Can you work these out from the model? Positions are in its coordinate system, mm. Face numbers are marked on the shaded views. Round coordinates to 2 decimals unless told otherwise and drop trailing zeros. Loops run counter-clockwise (first coordinate to the right, second up) from the corner with the lowest first, then second, coordinate; pieces in that order, holes last. Notation, with made-up numbers: (44, 22) -> (59, 22) arc R15 ccw to (59, 40) -> close; hole circle Ø9 at (-31, 39.5). An arc over 180 degrees is marked (long way). Write item = value, one per line.
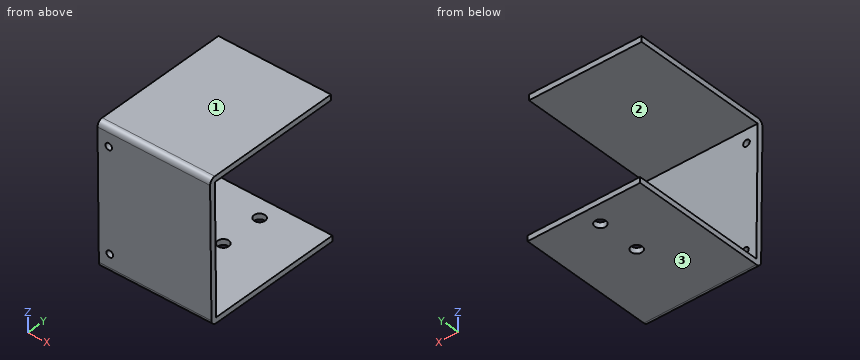
from build123d import *

# Parameters (mm, degrees)
F1_DEPTH = 50.8
F2_R     = 5
F3_DEPTH = 4.9999996097
F4_R     = 3
F5_DEPTH = 128.5401096596


with BuildPart() as f1:
    # F0 (on Right) → F1 (new body, symmetric)
    with BuildSketch(Plane.YZ):
        with BuildLine():
            Line((69.9766400008, 50.951808691), (69.9766400008, 55.9518083008))
            Line((69.9766400008, 55.9518083008), (-51.9620125118, 55.9518083008))
            ThreePointArc((-51.9620125118, 55.9518083008), (-55.5190376607, 54.4657195247), (-56.9616407497, 50.8908371368))
            Line((-56.9616407497, 50.8908371368), (-55.5349245808, -66.0997201058))
            ThreePointArc((-55.5349245808, -66.0997201058), (-54.0492075669, -69.5957740907), (-50.5352963429, -71.0387489418))
            Line((-50.5352963429, -71.0387489418), (71.525307565, -71.0387489418))
            Line((71.525307565, -71.0387489418), (71.525307565, -66.0387493321))
            Line((71.525307565, -66.0387493321), (-50.5352967284, -66.0387493321))
            Line((-50.5352967284, -66.0387493321), (-51.9620129069, 50.951808691))
            Line((-51.9620129069, 50.951808691), (69.9766400008, 50.951808691))
        make_face()
    extrude(amount=F1_DEPTH, both=True)

    # F2 (on face) → F3 (cut, through all)
    with BuildSketch(Plane(origin=(0, 0, -71.0387489418), x_dir=(1, 0, 0), z_dir=(0, 0, -1))):
        with Locations((0, -16)):
            Circle(F2_R)
        with Locations((0, -54.1)):
            Circle(F2_R)
    extrude(amount=-F3_DEPTH, mode=Mode.SUBTRACT)

    # F4 (on face) → F5 (cut, through all)
    with BuildSketch(Plane(origin=(0, -56.3326420192, -0.6869844294), x_dir=(1, 0, 0), z_dir=(0, -0.9999256476, -0.0121942328))):
        with Locations((-40.8, 39.5816567872)):
            Circle(F4_R)
        with Locations((-40.8, -53.4175996333)):
            Circle(F4_R)
    extrude(amount=-F5_DEPTH, mode=Mode.SUBTRACT)


solid = f1.part
1. I'm going to push flat-ended pins straight in: pin 1 (12 mm diameter, centred on x = 38.5, z = 39, fed in from -Y); pin 2 (4 mm diameter, centred on x = -21.5, z = 53, fed in from +Y); pin 3 (6 mm diameter, centred on x = -22, z = 5.5, fed in from -Y). Where does each tip first touch, or does it pass through?
Entries:
pin_1 = -56.89
pin_2 = 69.98
pin_3 = -56.44
2. Suppose I cut it at D-D, the plane x = -32. List the corners of the cut face in (y, z) for me.
Entries:
outline = (-56.96, 50.89) -> (-55.53, -66.1) arc R5 ccw to (-50.54, -71.04) -> (71.53, -71.04) -> (71.53, -66.04) -> (-50.54, -66.04) -> (-51.96, 50.95) -> (69.98, 50.95) -> (69.98, 55.95) -> (-51.96, 55.95) arc R5 ccw to start
3. Suppose I cut it at B-B, the plane y = -1. List the corners of the cut face in (x, z) for me.
Entries:
outline = (-50.8, -71.04) -> (50.8, -71.04) -> (50.8, -66.04) -> (-50.8, -66.04) -> close; (-50.8, 50.95) -> (50.8, 50.95) -> (50.8, 55.95) -> (-50.8, 55.95) -> close
4. I need wall thicknesses on line 1 (Z direction, x = 26, y = 14.5); line 2 (X direction, y = 16, z = -67.45); line 3 (Y direction, x = 0, z = -68). Which ranges of each line are inside material? Lowest first, please. Write a range as [from, to].
Entries:
line_1 = [-71.04, -66.04], [50.95, 55.95]
line_2 = [-50.8, -5], [5, 50.8]
line_3 = [-55.13, 11], [21, 49.1], [59.1, 71.53]
5. We'd pull the mould along Z, two halves only. Please class the marked faces 1, 2 and 3: released by +Z, released by -Z, zero draft, split by the parting line, or undercut.
Entries:
face_1 = released by +Z
face_2 = undercut
face_3 = released by -Z
6. Suppose I cut it at C-C, the plane y = 54.1. List the corners of the cut face in (x, z) for me.
Entries:
outline = (-50.8, -71.04) -> (-5, -71.04) -> (-5, -66.04) -> (-50.8, -66.04) -> close; (-50.8, 50.95) -> (50.8, 50.95) -> (50.8, 55.95) -> (-50.8, 55.95) -> close; (5, -71.04) -> (50.8, -71.04) -> (50.8, -66.04) -> (5, -66.04) -> close
7. Suppose I cut it at A-A, the plane x = 0. List the corners of the cut face in (y, z) for me, and give its area (3 significant figures).
Entries:
outline = (-56.96, 50.89) -> (-55.53, -66.1) arc R5 ccw to (-50.54, -71.04) -> (11, -71.04) -> (11, -66.04) -> (-50.54, -66.04) -> (-51.96, 50.95) -> (69.98, 50.95) -> (69.98, 55.95) -> (-51.96, 55.95) arc R5 ccw to start; (21, -71.04) -> (49.1, -71.04) -> (49.1, -66.04) -> (21, -66.04) -> close; (59.1, -71.04) -> (71.53, -71.04) -> (71.53, -66.04) -> (59.1, -66.04) -> close
area = 1,740 mm²
